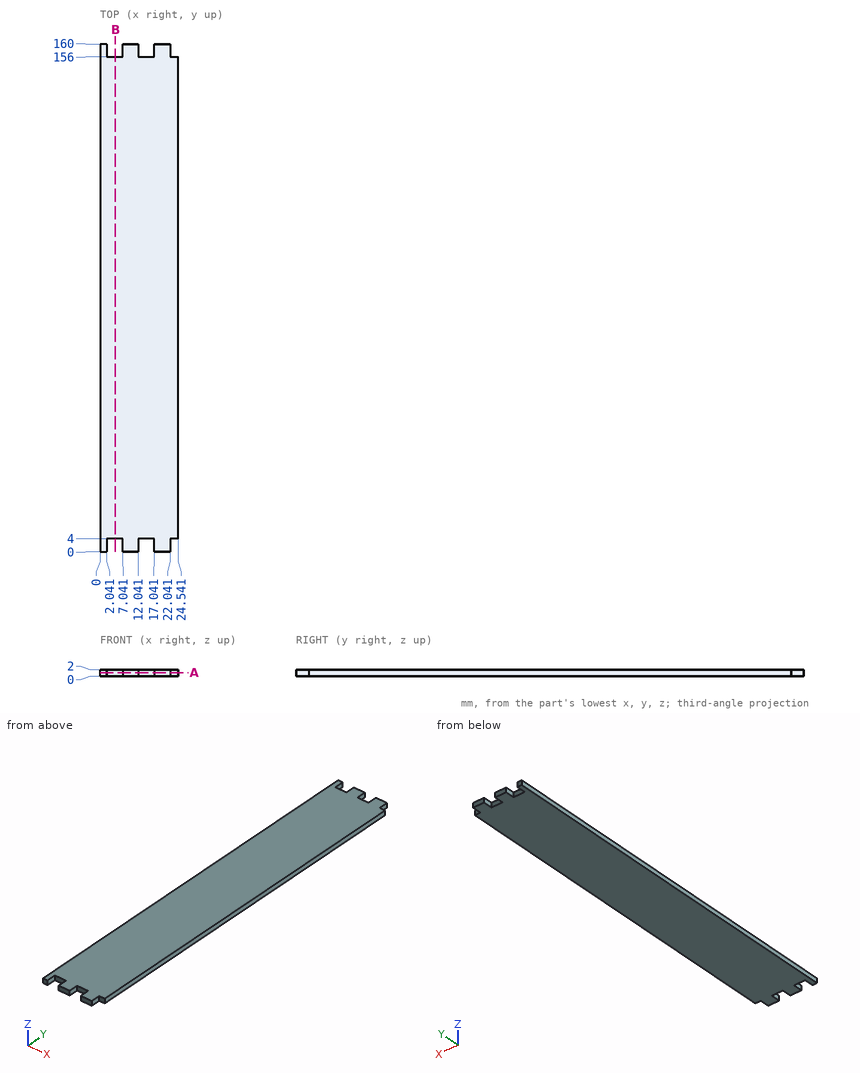
Verification items for this drawing (mm, ordinates from the low corner). Give positions to 0.01 mm unless a question says otherwise; leave off trailing zeros. Order: outer loops, then holes, each group sorted by start corner. A loop starts at its lowest first (then second) coordinate and runs counter-clockwise, first axis right, second up. Notation, with made-up numbers: M 6.25,24.5 L 32.25,24.5 A35 ccw 32.25,56.5 Z; hole C -34.75,71 d10. An arc over 180 degrees is marked long. Use a Markdown table: item, result.
Item 1: Section check B-B (x = 4.75). Record the cut outline in (y, z), and give its area (3 significant figures).
Answers follow:
| item | result |
|---|---|
| outline | M 4,0 L 156,0 L 156,2 L 4,2 Z |
| area | 304 mm2 |
Item 2: Depth check by flat-ended pin: P1, Ø0.6, axis at x = 14.5, z = 1.5, coming from the +Y side; P2, Ø0.6, axis at y = 1, z = 1, coming from the +X side; P3, Ø0.6, axis at x = 4, z = 1, coming from the -Y side. Enter the tip coordinate at first touch or a pass-through.
Answers follow:
| item | result |
|---|---|
| P1 | stops at y = 156 |
| P2 | stops at x = 22.04 |
| P3 | stops at y = 4 |
Item 3: Section check A-A (z = 1.1). Record the cut outline in (x, y).
Answers follow:
| item | result |
|---|---|
| outline | M 0,0 L 2.04,0 L 2.04,4 L 7.04,4 L 7.04,0 L 12.04,0 L 12.04,4 L 17.04,4 L 17.04,0 L 22.04,0 L 22.04,4 L 24.54,4 L 24.54,156 L 22.04,156 L 22.04,160 L 17.04,160 L 17.04,156 L 12.04,156 L 12.04,160 L 7.04,160 L 7.04,156 L 2.04,156 L 2.04,160 L 0,160 Z |
Item 4: Material ranges on line 1 along Y through (x, z) = (12.5, 0.3), recorded low to high.
Answers follow:
| item | result |
|---|---|
| line 1 | y = 4 to 156 |
